```python
from build123d import *

# Parameters (mm, degrees)
SKETCH1_W           = 19.05
SKETCH1_H           = 19.05
BOSS_EXTRUDE1_DEPTH = 44.45
BOSS_EXTRUDE2_DEPTH = 12.7
CUT_EXTRUDE1_DEPTH  = 45.45


with BuildPart() as part:
    # Sketch1 → Boss-Extrude1 (new body)
    with BuildSketch(Plane(origin=(0, 0, 0), x_dir=(1, 0, 0), z_dir=(0, 1, 0))):
        Rectangle(SKETCH1_W, SKETCH1_H)
    extrude(amount=BOSS_EXTRUDE1_DEPTH)

    # Sketch2 → Boss-Extrude2 (add)
    with BuildSketch(Plane(origin=(0, 44.45, 0), x_dir=(1, 0, 0), z_dir=(0, 1, 0))):
        Polygon((-9.525, -9.525), (-3.957241205, -9.525), (-9.525, -3.957241205), align=None)
    boss_extrude2 = extrude(amount=BOSS_EXTRUDE2_DEPTH)

    # Mirror1: Boss-Extrude2 across plane
    add(boss_extrude2.mirror(Plane(origin=(0, 0, 0), x_dir=(0.707106781, 0, 0.707106781), z_dir=(-0.707106781, 0, 0.707106781))))

    # Sketch3 → Cut-Extrude1 (cut, through all)
    with BuildSketch(Plane(origin=(0, 44.45, 0), x_dir=(1, 0, 0), z_dir=(0, 1, 0))):
        Polygon((9.525, -9.525), (-0.635, -9.525), (9.525, 0.635), align=None)
    cut_extrude1 = extrude(amount=-CUT_EXTRUDE1_DEPTH, mode=Mode.SUBTRACT)

    # Mirror2: Cut-Extrude1 across plane
    add(cut_extrude1.mirror(Plane(origin=(0, 0, 0), x_dir=(-0.707106781, 0, 0.707106781), z_dir=(-0.707106781, 0, -0.707106781))), mode=Mode.SUBTRACT)


solid = part.part
```
The model under review builds one solid part; all positions refer to its coordinate system, in mm. A direction names the side the tool comes from. Coordinates: 2 decimals unless noted, no trailing zeros. Write each loop counter-clockwise with the first axis right and the second up, starting at its lowest first coordinate (ties: lowest second). Pieces come first, ordered by that corner, then holes.
1) We need section B-B on z = -3. State the section outline as (x, y) points (3 decimals).
2) Clearance check with flat-ended pins moving along their axes: pin 1 Ø5 at (y, z) = (35, -6) entering from -X; pin 2 Ø4 at (x, z) = (6.5, -1) entering from -Y; pin 3 Ø5 at (y, z) = (30, -4) entering from -X; pin 4 Ø4 at (x, z) = (4.5, -6) entering from +Y. State where each tip first meets the part, or that it passes through.
3) To check wall thickness, follow probe 1 along Y at (x, z) = (1, 6.5); probe 2 along Z at (x, y) = (-7, 30) (3 decimals); probe 3 along Z at (x, y) = (2.75, 30.5) (3 decimals). State the ranges of each line that lie inside material, in increasing order.
4) We need section C-C on x = 8.25. State the section outline as (y, z) points (3 decimals), then the cut area to 3 significant figures.
5) We need section D-D on y = 42.5. State the section outline as (x, z) points (3 decimals).
6) Machinability: for faces 1 (the face through (6.78, 50.71, -6.7)), 2 (the face through (-6.7, 50.71, 6.78)), 3 (the face through (0, 44.45, 0)), which of the approach directions +Z, -Z, +X, -X, +Y, -Y give a long, thin tool a straight path to every point of the face, cutting with its end or side? Answer none if there is none.
7) We need section A-A on y = 49.5. State the section outline as (x, z) points (3 decimals).
Answer list:
1. outline: (-5.89, 0) - (9.525, 0) - (9.525, 44.45) - (-5.89, 44.45) - close
2. pin 1: stops at x = -5.39
2. pin 2: stops at y = 0
2. pin 3: stops at x = -7.39
2. pin 4: stops at y = 44.45
3. probe 1: y = 0 to 44.45
3. probe 2: z = -1.89 to 9.525
3. probe 3: z = -9.525 to 6.14
4. outline: (0, -9.525) - (57.15, -9.525) - (57.15, -5.232) - (44.45, -5.232) - (44.45, 0.64) - (0, 0.64) - close
4. area: 506 mm2
5. outline: (-9.525, 0.635) - (0.635, -9.525) - (9.525, -9.525) - (9.525, -0.635) - (-0.635, 9.525) - (-9.525, 9.525) - close
6. face 1: +Z, -X, +Y
6. face 2: -Z, +X, +Y
6. face 3: +Y
7. outline: (-9.525, 3.957) - (-3.957, 9.525) - (-9.525, 9.525) - close; (3.957, -9.525) - (9.525, -9.525) - (9.525, -3.957) - close
